Check sheet for the modelled part. Datum: model origin and axes. Units: mm. A direction names the side the tool comes from. Round coordinates to 2 decimals unless told otherwise and drop trailing zeros. Loops run counter-clockwise (first coordinate to the right, second up) from the corner with the lowest first, then second, coordinate; pieces in that order, holes last. Notation, with made-up numbers: M 20.25,53.5 L 40.25,53.5 A24 ccw 40.25,69.5 Z; hole C 32.25,41.5 d6. An arc over 180 degrees is marked long. One line per question, with ' | ' between items. Start each with the question number.
(1) Go/stop test with flat-tipped pins: P1, Ø2, axis at x = 33.5, z = 4.5, coming from the +Y side; P2, Ø1, axis at y = 2, z = 2, coming from the +X side; P3, Ø4, axis at x = 73.44, y = 85.2, coming from the -Z side; P4, Ø1.5, axis at x = -122, z = 3, coming from the +Y side. Record where each tip stops, or that it passes through.
(2) Thickness scan on probe 1 along Y at (x, z) = (21, 4); probe 2 along X at (y, z) = (107.5, 4.45); probe 3 along Y at (x, z) = (23, 2.25). Record the ranges inside material, lowest first. Write a range as [from, to].
(3) Section check A-A (z = 3.15). Count the separate pieces of the cut face and the enclosed holes in it, and give its area (3 significant figures).
(4) Section check B-B (x = -16). Record the boundary of the cut face in (y, z), and give its area (3 significant figures).
(5) Draft check along X on faces 3 (the face through (-95, 0, 2)), 4 (the face through (-3.179, 100.945, 2.465)), 5 (the face through (6, 2, 5)). Enter one of: +X half, -X half, draft (parallel to the pull), parting line (faces both ways), or undercut.
(6) Tool access check on faces 1 (the face through (-132.59, 27.94, 2.46)), 2 (the face through (-82.163, -34.209, 2.535)). Record the directions out of +Z, -Z, +X, -X, +Y, -Y that give a thin tool (end or side, any length) a straight path to the whole face; none if there is none.
```python
from build123d import *

# Parameters (mm, degrees)
SKETCH1_R           = 4.025
SKETCH1_R_2         = 1.65
SKETCH1_R_3         = 2
SKETCH1_R_4         = 3
SKETCH1_W           = 9
SKETCH1_H           = 15
BOSS_EXTRUDE1_DEPTH = 5
CUT_EXTRUDE1_DEPTH  = 186.946581396
SKETCH3_R           = 1.4
CUT_EXTRUDE2_DEPTH  = 186.946581396
CUT_EXTRUDE4_DEPTH  = 186.946581396
CIRPATTERN1_COUNT   = 3


with BuildPart() as part:
    # Sketch1 → Boss-Extrude1 (new body)
    with BuildSketch(Plane.XY):
        with BuildLine():
            Line((-127.0125, 29.449853865), (38.001928415, 124.720978531))
            Line((38.001928415, 124.720978531), (36.501939089, 127.319036255))
            ThreePointArc((36.501939089, 127.319036255), (42.014428415, 128.796103318), (47.526917741, 127.319036255))
            Line((47.526917741, 127.319036255), (86.498060911, 104.819036255))
            ThreePointArc((86.498060911, 104.819036255), (90.533483174, 100.783613992), (92.010550238, 95.271124665))
            Line((92.010550238, 95.271124665), (89.010571585, 95.271124665))
            Line((89.010571585, 95.271124665), (89.010571585, -95.271124665))
            Line((89.010571585, -95.271124665), (92.010550238, -95.271124665))
            ThreePointArc((92.010550238, -95.271124665), (90.671767887, -100.536839764), (86.980562177, -104.523704959))
            Line((86.980562177, -104.523704959), (47.529952044, -127.317283756))
            ThreePointArc((47.529952044, -127.317283756), (42.016179814, -128.796103179), (36.501938019, -127.319035637))
            Line((36.501938019, -127.319035637), (38.001927636, -124.720978081))
            Line((38.001927636, -124.720978081), (-127.012490105, -29.449834928))
            Line((-127.012490105, -29.449834928), (-128.512490396, -32.047910972))
            ThreePointArc((-128.512490396, -32.047910972), (-132.547911898, -28.012488791), (-134.024978652, -22.5))
            Line((-134.024978652, -22.5), (-134.024978652, 22.5))
            ThreePointArc((-134.024978652, 22.5), (-132.547911589, 28.012489326), (-128.512489326, 32.047911589))
            Line((-128.512489326, 32.047911589), (-127.0125, 29.449853865))
        make_face()
        with Locations((-123, 22.5)):
            Circle(SKETCH1_R, mode=Mode.SUBTRACT)
        with Locations((-123, -22.5)):
            Circle(SKETCH1_R, mode=Mode.SUBTRACT)
        with Locations((42.014428415, 117.771124665)):
            Circle(SKETCH1_R, mode=Mode.SUBTRACT)
        with Locations((80.985571585, 95.271124665)):
            Circle(SKETCH1_R, mode=Mode.SUBTRACT)
        with Locations((80.985571585, -95.271124665)):
            Circle(SKETCH1_R, mode=Mode.SUBTRACT)
        with Locations((42.014428415, -117.771124665)):
            Circle(SKETCH1_R, mode=Mode.SUBTRACT)
        with Locations((-110.5, 21)):
            Circle(SKETCH1_R_2, mode=Mode.SUBTRACT)
        with Locations((-110.5, -21)):
            Circle(SKETCH1_R_2, mode=Mode.SUBTRACT)
        with Locations((73.436533479, 85.195807118)):
            Circle(SKETCH1_R_2, mode=Mode.SUBTRACT)
        with Locations((37.063466521, 106.195807118)):
            Circle(SKETCH1_R_2, mode=Mode.SUBTRACT)
        with Locations((37.063466521, -106.195807118)):
            Circle(SKETCH1_R_2, mode=Mode.SUBTRACT)
        with Locations((73.436533479, -85.195807118)):
            Circle(SKETCH1_R_2, mode=Mode.SUBTRACT)
        Circle(SKETCH1_R_3, mode=Mode.SUBTRACT)
        with Locations((-92, 0)):
            Circle(SKETCH1_R_4, mode=Mode.SUBTRACT)
        with Locations((46, 79.674337148)):
            Circle(SKETCH1_R_4, mode=Mode.SUBTRACT)
        with Locations((46, -79.674337148)):
            Circle(SKETCH1_R_4, mode=Mode.SUBTRACT)
        Polygon((70.245190528, 106.668238983), (65.745190528, 98.874010348), (52.754809472, 106.374010348), (57.254809472, 114.168238983), align=None, mode=Mode.SUBTRACT)
        with Locations((-123, 0)):
            Rectangle(SKETCH1_W, SKETCH1_H, mode=Mode.SUBTRACT)
        Polygon((57.254809472, -114.168238983), (52.754809472, -106.374010348), (65.745190528, -98.874010348), (70.245190528, -106.668238983), align=None, mode=Mode.SUBTRACT)
    extrude(amount=BOSS_EXTRUDE1_DEPTH)

    # Sketch2 → Cut-Extrude1 (cut, through all)
    with BuildSketch(Plane.XY.offset(5)):
        Polygon((89.010571585, 1.48), (80.010571585, 1.48), (80.010571585, 3.5), (79.510571585, 3.5), (79.510571585, 2.75), (77.010571585, 2.75), (77.010571585, 1.48), (75.010571585, 1.48), (75.010571585, -1.48), (77.010571585, -1.48), (77.010571585, -2.75), (79.510571585, -2.75), (79.510571585, -3.5), (80.010571585, -3.5), (80.010571585, -1.48), (89.010571585, -1.48), align=None)
        Polygon((-43.223568195, -77.825416198), (-38.723568195, -70.031187564), (-36.974196879, -71.041187564), (-36.724196879, -70.608174862), (-37.373715932, -70.233174862), (-36.123715932, -68.068111353), (-37.223568195, -67.433111353), (-36.223568195, -65.701060545), (-38.78700339, -64.221060545), (-39.78700339, -65.953111353), (-40.886855653, -65.318111353), (-42.136855653, -67.483174862), (-42.786374706, -67.108174862), (-43.036374706, -67.541187564), (-41.28700339, -68.551187564), (-45.78700339, -76.345416198), align=None)
        Polygon((-45.78700339, 76.345416198), (-41.28700339, 68.551187564), (-43.036374706, 67.541187564), (-42.786374706, 67.108174862), (-42.136855653, 67.483174862), (-40.886855653, 65.318111353), (-39.78700339, 65.953111353), (-38.78700339, 64.221060545), (-36.223568195, 65.701060545), (-37.223568195, 67.433111353), (-36.123715932, 68.068111353), (-37.373715932, 70.233174862), (-36.724196879, 70.608174862), (-36.974196879, 71.041187564), (-38.723568195, 70.031187564), (-43.223568195, 77.825416198), align=None)
    extrude(amount=-CUT_EXTRUDE1_DEPTH, mode=Mode.SUBTRACT)

    # Sketch3 → Cut-Extrude2 (cut, through all)
    with BuildSketch(Plane.XY.offset(5)):
        with Locations((-82.342452032, -50.621297655)):
            Circle(SKETCH3_R)
        with Locations((-2.668120037, -96.621306581)):
            Circle(SKETCH3_R)
        with Locations((54.831891121, 2.971608412)):
            Circle(SKETCH3_R)
        with Locations((-24.842440874, 48.971617338)):
            Circle(SKETCH3_R)
        with BuildLine():
            Line((-110.290058805, -34.485735187), (-98.165703936, -41.485736545))
            ThreePointArc((-98.165703936, -41.485736545), (-97.406884902, -41.585637053), (-96.799678491, -41.119711294))
            Line((-96.799678491, -41.119711294), (-92.799677715, -34.191508512))
            ThreePointArc((-92.799677715, -34.191508512), (-92.699777207, -33.432689478), (-93.165702966, -32.825483067))
            Line((-93.165702966, -32.825483067), (-105.290057834, -25.825481709))
            ThreePointArc((-105.290057834, -25.825481709), (-106.048876868, -25.725581202), (-106.656083279, -26.19150696))
            Line((-106.656083279, -26.19150696), (-110.656084055, -33.119709742))
            ThreePointArc((-110.656084055, -33.119709742), (-110.755984563, -33.878528776), (-110.290058805, -34.485735187))
        make_face()
    extrude(amount=-CUT_EXTRUDE2_DEPTH, mode=Mode.SUBTRACT)

    # Sketch6 → Cut-Extrude4 (cut, through all)
    with BuildSketch(Plane.XY.offset(5)):
        with BuildLine():
            ThreePointArc((-77.076260937, 44.5), (-82.225278394, 34.05882548), (-85.96739854, 23.034895014))
            ThreePointArc((-85.96739854, 23.034895014), (-84.553184977, 20.585405271), (-82.103695235, 21.999618834))
            ThreePointArc((-82.103695235, 21.999618834), (-78.529760263, 32.528091751), (-73.612159322, 42.5))
            ThreePointArc((-73.612159322, 42.5), (-74.344210129, 45.232050808), (-77.076260937, 44.5))
        make_face()
        with BuildLine():
            ThreePointArc((-73.612159322, -42.5), (-74.344210129, -45.232050808), (-77.076260937, -44.5))
            ThreePointArc((-77.076260937, -44.5), (-82.225278394, -34.05882548), (-85.96739854, -23.034895014))
            ThreePointArc((-85.96739854, -23.034895014), (-84.553184977, -20.585405271), (-82.103695235, -21.999618834))
            ThreePointArc((-82.103695235, -21.999618834), (-78.529760263, -32.528091751), (-73.612159322, -42.5))
        make_face()
    cut_extrude4 = extrude(amount=-CUT_EXTRUDE4_DEPTH, mode=Mode.SUBTRACT)

    # CirPattern1: Cut-Extrude4 ×3 about axis
    cirpattern1_axis = Axis((0, 0, 0), (0, 0, 1))
    for i in range(1, CIRPATTERN1_COUNT):
        add(cut_extrude4.rotate(cirpattern1_axis, i * 360 / CIRPATTERN1_COUNT), mode=Mode.SUBTRACT)


solid = part.part
```
The answers:
1) P1: y = 122.7 | P2: x = 89.01 | P3: z = 0 | P4: y = 32.78
2) probe 1: [-114.9, -86.49], [-82.37, 82.37], [86.49, 114.9] | probe 2: [8.17, 36.05], [38.07, 53.4], [68.8, 81.85] | probe 3: [-116.06, -85.98], [-82.09, 82.09], [85.98, 116.06]
3) separate pieces: 1 | enclosed holes: 30 | area: 36,100 mm²
4) outline: M -93.54,0 L 93.54,0 L 93.54,5 L -93.54,5 Z | area: 935 mm²
5) face 3: undercut | face 4: -X half | face 5: draft
6) face 1: +Z, -Z, -X, +Y | face 2: +Z, -Z
